```python
from build123d import *

# Parameters (mm, degrees)
SKETCH_1_W           = 280
SKETCH_1_H           = 280
EXTRUDE_1_DEPTH      = 5
SKETCH_2_R           = 80
CUT_EXTRUDE_1_DEPTH  = 5
SKETCH_3_W           = 20
SKETCH_3_H           = 43
EXTRUDE_2_DEPTH      = 45
SKETCH_4_R           = 11
CUT_EXTRUDE_2_DEPTH  = 400.12404087
SKETCH_5_R           = 16.2
CUT_EXTRUDE_3_DEPTH  = 7.2
CUT_EXTRUDE_START    = -7.2
SKETCH_6_R           = 16.2
CUT_EXTRUDE_4_DEPTH  = 7.2
SKETCH_7_R           = 16.2
CUT_EXTRUDE_5_DEPTH  = 7.2
SKETCH_8_R           = 16.2
CUT_EXTRUDE_6_DEPTH  = 7.2
SKETCH_9_W           = 280
SKETCH_9_H           = 80
CUT_EXTRUDE_7_DEPTH  = 399.52854352
CHAMFER_1_SIZE       = 70
FILLET_1_R           = 21.5
FILLET_2_R           = 12
FILLET_3_R           = 2
SKETCH_10_R          = 1.6
CUT_EXTRUDE_8_DEPTH  = 5
SKETCH_11_R          = 2.35
CUT_EXTRUDE_9_DEPTH  = 4.2
CHAMFER_4_SIZE       = 0.4
SKETCH_12_R          = 1.65
CUT_EXTRUDE_10_DEPTH = 10
SKETCH_13_R          = 2.9
CUT_EXTRUDE_11_DEPTH = 2.5


with BuildPart() as part:
    # 草图1 → 凸台-拉伸1 (new body)
    with BuildSketch(Plane(origin=(0, 0, 0), x_dir=(1, 0, 0), z_dir=(0, 1, 0))):
        with Locations((140, -140)):
            Rectangle(SKETCH_1_W, SKETCH_1_H)
    extrude(amount=EXTRUDE_1_DEPTH)

    # 草图2 → 切除-拉伸1 (cut)
    with BuildSketch(Plane(origin=(0, 5, 0), x_dir=(1, 0, 0), z_dir=(0, 1, 0))):
        with Locations(Location((140, -180, 0), (0, 0, 270))):
            Circle(SKETCH_2_R)
    extrude(amount=-CUT_EXTRUDE_1_DEPTH, mode=Mode.SUBTRACT)

    # 草图3 → 凸台-拉伸2 (add)
    with BuildSketch(Plane(origin=(0, 5, 0), x_dir=(1, 0, 0), z_dir=(0, 1, 0))):
        with Locations((10, -180)):
            Rectangle(SKETCH_3_W, SKETCH_3_H)
        with Locations((270, -180)):
            Rectangle(SKETCH_3_W, SKETCH_3_H)
    extrude(amount=EXTRUDE_2_DEPTH)

    # 草图4 → 切除-拉伸2 (cut, through all)
    with BuildSketch(Plane(origin=(280, 0, 0), x_dir=(0, 0, -1), z_dir=(1, 0, 0))):
        with Locations((-180, 30)):
            Circle(SKETCH_4_R)
    extrude(amount=-CUT_EXTRUDE_2_DEPTH, mode=Mode.SUBTRACT)

    # 草图5 → 切除-拉伸3 (cut)
    with BuildSketch(Plane(origin=(280, 0, 0), x_dir=(0, 0, -1), z_dir=(1, 0, 0))):
        with Locations((-180, 30)):
            Circle(SKETCH_5_R)
    extrude(amount=-CUT_EXTRUDE_3_DEPTH, mode=Mode.SUBTRACT)

    # 草图6 → 切除-拉伸4 (cut)
    with BuildSketch(Plane.ZY.offset(-260).offset(CUT_EXTRUDE_START)):
        with Locations(Location((180, 30, 0), (0, 0, 180))):
            Circle(SKETCH_6_R)
    extrude(amount=CUT_EXTRUDE_4_DEPTH, mode=Mode.SUBTRACT)

    # 草图7 → 切除-拉伸5 (cut)
    with BuildSketch(Plane(origin=(20, 0, 0), x_dir=(0, 0, -1), z_dir=(1, 0, 0))):
        with Locations((-180, 30)):
            Circle(SKETCH_7_R)
    extrude(amount=-CUT_EXTRUDE_5_DEPTH, mode=Mode.SUBTRACT)

    # 草图8 → 切除-拉伸6 (cut)
    with BuildSketch(Plane.ZY.offset(CUT_EXTRUDE_START)):
        with Locations(Location((180, 30, 0), (0, 0, 180))):
            Circle(SKETCH_8_R)
    extrude(amount=CUT_EXTRUDE_6_DEPTH, mode=Mode.SUBTRACT)

    # 草图9 → 切除-拉伸7 (cut, through all)
    with BuildSketch(Plane(origin=(0, 5, 0), x_dir=(1, 0, 0), z_dir=(0, 1, 0))):
        with Locations((140, -40)):
            Rectangle(SKETCH_9_W, SKETCH_9_H)
    extrude(amount=-CUT_EXTRUDE_7_DEPTH, mode=Mode.SUBTRACT)

    # 倒角1
    chamfer_1_edges = [part.edges().sort_by_distance(p)[0] for p in [
        (280, 2.5, 280),
        (0, 2.5, 280),
        (0, 2.5, 80),
        (280, 2.5, 80),
    ]]
    chamfer(chamfer_1_edges, length=CHAMFER_1_SIZE)

    # 圆角1
    fillet_1_edges = [part.edges().sort_by_distance(p)[0] for p in [
        (270, 50, 201.5),
        (270, 50, 158.5),
        (10, 50, 201.5),
        (10, 50, 158.5),
    ]]
    fillet(fillet_1_edges, radius=FILLET_1_R - 0.0001)  # a hair under: the kernel refuses the full size

    # 圆角2
    fillet_2_edges = [part.edges().sort_by_distance(p)[0] for p in [
        (280, 2.5, 210),
        (280, 2.5, 150),
        (70, 2.5, 80),
        (210, 2.5, 80),
        (70, 2.5, 280),
        (210, 2.5, 280),
        (0, 2.5, 150),
        (0, 2.5, 210),
    ]]
    fillet(fillet_2_edges, radius=FILLET_2_R)

    # 圆角3
    fillet_3_edges = [part.edges().sort_by_distance(p)[0] for p in [
        (10, 5, 201.5),
        (20, 5, 180),
        (10, 5, 158.5),
        (270, 5, 158.5),
        (260, 5, 180),
        (270, 5, 201.5),
    ]]
    fillet(fillet_3_edges, radius=FILLET_3_R)

    # 草图10 → 切除-拉伸8 (cut)
    with BuildSketch(Plane(origin=(0, 0, 0), x_dir=(-1, 0, 0), z_dir=(0, -1, 0))):
        with Locations(Location((-20, -187.5, 0), (0, 0, 90))):
            Circle(SKETCH_10_R)
        with Locations(Location((-20, -172.5, 0), (0, 0, 90))):
            Circle(SKETCH_10_R)
        with Locations(Location((-260, -187.5, 0), (0, 0, 270))):
            Circle(SKETCH_10_R)
        with Locations(Location((-260, -172.5, 0), (0, 0, 270))):
            Circle(SKETCH_10_R)
    extrude(amount=-CUT_EXTRUDE_8_DEPTH, mode=Mode.SUBTRACT)

    # 草图11 → 切除-拉伸9 (cut)
    with BuildSketch(Plane(origin=(0, 0, 0), x_dir=(-1, 0, 0), z_dir=(0, -1, 0))):
        with Locations(Location((-20, -172.5, 0), (0, 0, 90))):
            Circle(SKETCH_11_R)
        with Locations(Location((-20, -187.5, 0), (0, 0, 90))):
            Circle(SKETCH_11_R)
        with Locations(Location((-260, -172.5, 0), (0, 0, 90))):
            Circle(SKETCH_11_R)
        with Locations(Location((-260, -187.5, 0), (0, 0, 90))):
            Circle(SKETCH_11_R)
    extrude(amount=-CUT_EXTRUDE_9_DEPTH, mode=Mode.SUBTRACT)

    # 倒角4
    chamfer_4_edges = [part.edges().sort_by_distance(p)[0] for p in [
        (140, 0, 80),
        (140, 0, 100),
        (35, 0, 115),
        (245, 0, 115),
        (280, 0, 180),
        (245, 0, 245),
        (140, 0, 280),
        (35, 0, 245),
        (0, 0, 180),
        (0.91344561, 0, 150.37836156),
        (0.91344561, 0, 209.62163844),
        (70.37836156, 0, 279.08655439),
        (209.62163844, 0, 279.08655439),
        (279.08655439, 0, 209.62163844),
        (279.08655439, 0, 150.37836156),
        (209.62163844, 0, 80.91344561),
        (70.37836156, 0, 80.91344561),
        (20, 0, 189.85),
        (260, 0, 174.85),
        (260, 0, 189.85),
        (20, 0, 174.85),
    ]]
    chamfer(chamfer_4_edges, length=CHAMFER_4_SIZE)

    # 草图12 → 切除-拉伸10 (cut)
    with BuildSketch(Plane(origin=(0, 5, 0), x_dir=(1, 0, 0), z_dir=(0, 1, 0))):
        with Locations(Location((118.5, -85, 0), (0, 0, 270))):
            Circle(SKETCH_12_R)
        with Locations(Location((161.5, -85, 0), (0, 0, 270))):
            Circle(SKETCH_12_R)
    extrude(amount=-CUT_EXTRUDE_10_DEPTH, mode=Mode.SUBTRACT)

    # 草图13 → 切除-拉伸11 (cut)
    with BuildSketch(Plane(origin=(0, 5, 0), x_dir=(1, 0, 0), z_dir=(0, 1, 0))):
        with Locations(Location((118.5, -85, 0), (0, 0, 270))):
            Circle(SKETCH_13_R)
        with Locations(Location((161.5, -85, 0), (0, 0, 270))):
            Circle(SKETCH_13_R)
    extrude(amount=-CUT_EXTRUDE_11_DEPTH, mode=Mode.SUBTRACT)


solid = part.part
```
Check sheet for the modelled part. Datum: model origin and axes. Units: mm. A direction names the side the tool comes from. Coordinates: 2 decimals unless noted, no trailing zeros. Write each loop counter-clockwise with the first axis right and the second up, starting at its lowest first coordinate (ties: lowest second). Pieces come first, ordered by that corner, then holes. Notation, with made-up numbers: (61.25, 85) - (112.25, 85) arc R15 ccw to (112.25, 104) - close; hole circle Ø2 at (37.5, -31). An arc over 180 degrees is marked (long way). One line per question, with ' | ' between items.
Item 1: Mould release check, pull along Y, two halves, no side actions. Record for faces 1 (the face through (270, 30, 191)), 2 (the face through (159.735, 3.768, 82.699)), 3 (the face through (34.7, 0.2, 115.58)): pulls with the +Y half, pulls with the -Y half, needs draft (parallel to the pull), parting line crosses it, or undercut.
Determined:
face 1: undercut | face 2: needs draft | face 3: pulls with the -Y half
Item 2: Sectioned sample at C-C on x = 50.5. Record the boundary of the cut face in (y, z).
Determined:
outline: (0, 100.07) - (0.4, 99.5) - (5, 99.5) - (5, 260.5) - (0.4, 260.5) - (0, 259.93) - close
Item 3: Sectioned sample at B-B on y = 22. Give the number of separate pieces and of enclosed holes in the cut face, plus the area to 3 significant figures.
Determined:
separate pieces: 4 | enclosed holes: 0 | area: 739 mm2
Item 4: Gauge pin test, flat ends, axial feed: P1, Ø4, axis at x = 20, z = 172.5, coming from the +Y side; P2, Ø6, axis at x = 69.5, y = 7, coming from the +Z side; P3, Ø1.4, axis at x = 259, z = 172, coming from the -Y side. Record the tip position at first contact, or that the pin passes through.
Determined:
P1: stops at y = 49.28 | P2: stops at z = 279.56 | P3: stops at y = 4.2
Item 5: Sectioned sample at D-D on z = 265.5. Record the boundary of the cut face in (x, y).
Determined:
outline: (55.5, 0.4) - (56.07, 0) - (223.93, 0) - (224.5, 0.4) - (224.5, 5) - (55.5, 5) - close
Item 6: Thickness scan on line 1 (Z direction, x = 260, y = 4); line 2 (X direction, y = 8, z = 199); line 3 (X direction, y = 2, z = 180). Record the ranges inside material, lowest first. Write a range as [from, to].
Determined:
line 1: z = [130, 170.15], [174.85, 185.15], [189.85, 230] | line 2: x = [0, 20], [260, 280] | line 3: x = [0, 60], [220, 280]
Item 7: Sectioned sample at A-A on x = 140. Record the boundary of the cut face in (y, z), plus the area to 3 significant figures.
Determined:
outline: (0, 80.4) - (0.4, 80) - (5, 80) - (5, 100) - (0.4, 100) - (0, 99.6) - close; (0, 260.4) - (0.4, 260) - (5, 260) - (5, 280) - (0.4, 280) - (0, 279.6) - close | area: 200 mm2
Item 8: Access from +Z, -Z, +X, -X, +Y, -Y to the whole of each face (thin tool, end or side, straight path). Record for faces 4 (the face through (7.2, 33, 169)), 5 (the face through (276.45, 40.95, 191.94)), 6 (the face through (16.45, 40.95, 191.94)).
Determined:
face 4: -X | face 5: +X | face 6: none
